```python
from build123d import *

# Parameters (mm, degrees)
EXTRUDE_1_DEPTH        = 500
SKETCH_2_R             = 3
SKETCH_2_R_2           = 1.75
CUT_EXTRUDE_1_DEPTH    = 4.5
SKETCH_2_2_R           = 1.75
CUT_EXTRUDE_2_DEPTH    = 9
PATTERN_LINEAR_1_COUNT = 20
PATTERN_LINEAR_1_PITCH = 25


with BuildPart() as part:
    # Эскиз1 → Бобышка-Вытянуть1 (new body)
    with BuildSketch(Plane.XY):
        with BuildLine():
            Line((-6, 3.7), (-5.7, 4))
            Line((-5.7, 4), (5.7, 4))
            Line((5.7, 4), (6, 3.7))
            Line((6, 3.7), (6, 2.451013544))
            ThreePointArc((6, 2.451013544), (5.597935912, 2.202976267), (5.354599002, 1.798050138))
            Line((5.354599002, 1.798050138), (4.643514056, 1.798050138))
            Line((4.643514056, 1.798050138), (4.643514056, 1.201949862))
            Line((4.643514056, 1.201949862), (5.354599002, 1.201949862))
            ThreePointArc((5.354599002, 1.201949862), (5.597935912, 0.797023733), (6, 0.548986456))
            Line((6, 0.548986456), (6, -3.7))
            Line((6, -3.7), (5.7, -4))
            Line((5.7, -4), (-5.7, -4))
            Line((-5.7, -4), (-6, -3.7))
            Line((-6, -3.7), (-6, 0.548986456))
            ThreePointArc((-6, 0.548986456), (-5.597935912, 0.797023733), (-5.354599002, 1.201949862))
            Line((-5.354599002, 1.201949862), (-4.643514056, 1.201949862))
            Line((-4.643514056, 1.201949862), (-4.643514056, 1.798050138))
            Line((-4.643514056, 1.798050138), (-5.354599002, 1.798050138))
            ThreePointArc((-5.354599002, 1.798050138), (-5.597935912, 2.202976267), (-6, 2.451013544))
            Line((-6, 2.451013544), (-6, 3.7))
        make_face()
    extrude(amount=EXTRUDE_1_DEPTH)

    # Эскиз2 → Вырез-Вытянуть1 (cut)
    with BuildSketch(Plane(origin=(0, 4, 0), x_dir=(1, 0, 0), z_dir=(0, 1, 0))):
        with Locations((0, -12)):
            Circle(SKETCH_2_R)
        with Locations((0, -12)):
            Circle(SKETCH_2_R_2, mode=Mode.SUBTRACT)
    cut_extrude_1 = extrude(amount=-CUT_EXTRUDE_1_DEPTH, mode=Mode.SUBTRACT)

    # Эскиз2<2> → Вырез-Вытянуть2 (cut, through all)
    with BuildSketch(Plane(origin=(0, 4, 0), x_dir=(1, 0, 0), z_dir=(0, 1, 0))):
        with Locations((0, -12)):
            Circle(SKETCH_2_2_R)
    cut_extrude_2 = extrude(amount=-CUT_EXTRUDE_2_DEPTH, mode=Mode.SUBTRACT)

    # Линейный массив1: Вырез-Вытянуть1, Вырез-Вытянуть2 ×20
    with Locations(*[(0, 0, i * PATTERN_LINEAR_1_PITCH) for i in range(1, PATTERN_LINEAR_1_COUNT)]):
        add(cut_extrude_1, mode=Mode.SUBTRACT)
        add(cut_extrude_2, mode=Mode.SUBTRACT)


solid = part.part
```
Build history of the part. All positions in model axes, mm. Coordinates: 2 decimals unless noted, no trailing zeros.
Item 1: Drill centre lines: L1, parallel to X at y = 2.9, z = 137; L2, parallel to X at y = 1.25, z = 262; L3, parallel to Y at x = -5, z = 339. Where is each one in solid material? Low to high.
Filled in:
L1: x = -6 to -3, 3 to 6
L2: x = -4.64 to -3, 3 to 4.64
L3: y = -4 to 1.2, 1.8 to 4
Item 2: Saw through at A-A on y = -2.5. State how many separate pieces and enclosed holes the cut face has, then the cut area to 3 significant figures.
Filled in:
separate pieces: 1
enclosed holes: 20
area: 5,810 mm2
Item 3: Drop flat-ended pins along their axis: pin 1 Ø1.8 at (x, z) = (-1, 63.5) entering from +Y; pin 2 Ø1 at (y, z) = (1.5, 146) entering from -X. Give the stop position or say it passes through.
Filled in:
pin 1: stops at y = -0.5
pin 2: stops at x = -5.44
